```python
from build123d import *

# Parameters (mm, degrees)
EXTRUDE_1_DEPTH     = 900
CUT_EXTRUDE_1_DEPTH = 40


with BuildPart() as part:
    # Эскиз1 → Вытянуть-Тонкостенный1 (new body)
    with BuildSketch(Plane(origin=(0, 0, 0), x_dir=(0, 0, -1), z_dir=(1, 0, 0))):
        with BuildLine():
            Line((-3, 53), (-3, 1))
            ThreePointArc((-3, 1), (-1.828427125, -1.828427125), (1, -3))
            Line((1, -3), (33, -3))
            ThreePointArc((33, -3), (35.828427125, -1.828427125), (37, 1))
            Line((37, 1), (37, 53))
            ThreePointArc((37, 53), (35.828427125, 55.828427125), (33, 57))
            Line((33, 57), (1, 57))
            ThreePointArc((1, 57), (-1.828427125, 55.828427125), (-3, 53))
        make_face()
        with BuildLine():
            Line((0, 53), (0, 1))
            ThreePointArc((0, 1), (0.292893219, 0.292893219), (1, 0))
            Line((1, 0), (33, 0))
            ThreePointArc((33, 0), (33.707106781, 0.292893219), (34, 1))
            Line((34, 1), (34, 53))
            ThreePointArc((34, 53), (33.707106781, 53.707106781), (33, 54))
            Line((33, 54), (1, 54))
            ThreePointArc((1, 54), (0.292893219, 53.707106781), (0, 53))
        make_face(mode=Mode.SUBTRACT)
    extrude(amount=EXTRUDE_1_DEPTH)

    # Эскиз2 → Вырез-Вытянуть1 (cut)
    with BuildSketch(Plane.XY.offset(3)):
        with BuildLine():
            Line((20, 32), (50, 32))
            ThreePointArc((50, 32), (55, 27), (50, 22))
            Line((50, 22), (20, 22))
            ThreePointArc((20, 22), (15, 27), (20, 32))
        make_face()
    extrude(amount=-CUT_EXTRUDE_1_DEPTH, mode=Mode.SUBTRACT)


solid = part.part
```
Geometry: final body of the model. Coordinates: model frame, mm. A direction names the side the tool comes from. Coordinates: 2 decimals unless noted, no trailing zeros. Order: outer loops, then holes, each group sorted by start corner. A loop starts at its lowest first (then second) coordinate and runs counter-clockwise, first axis right, second up. Notation, with made-up numbers: (63.25, -4) - (88.25, -4) arc R33 cw to (88.25, 25) - close; hole circle Ø8 at (-38.5, 70.5). An arc over 180 degrees is marked (long way). Write each question's results on one line, items separated by ' | '.
(1) Set-up query: faces 4 (the face through (444, 27, 0)), 5 (the face through (444, 27, 3)). Return all of +Z, -Z, +X, -X, +Y, -Y with unobstructed straight access to the full face (end or side cutting, diameter ignored); none if empty.
Values found:
face 4: +X, -X | face 5: +Z, +X, -X, +Y, -Y
(2) Section query B-B, the plane z = -14. Return the cut outline in (x, y), plus the area to 3 significant figures.
Values found:
outline: (0, -3) - (900, -3) - (900, 0) - (0, 0) - close; (0, 54) - (900, 54) - (900, 57) - (0, 57) - close | area: 5,400 mm²
(3) Section query C-C, the plane x = 818.5. Return the cut outline in (y, z), plus the area to 3 significant figures.
Values found:
outline: (-3, -33) arc R4 ccw to (1, -37) - (53, -37) arc R4 ccw to (57, -33) - (57, -1) arc R4 ccw to (53, 3) - (1, 3) arc R4 ccw to (-3, -1) - close; hole (0, -33) arc R1 ccw to (1, -34) - (53, -34) arc R1 ccw to (54, -33) - (54, -1) arc R1 ccw to (53, 0) - (1, 0) arc R1 ccw to (0, -1) - close | area: 551 mm²
(4) First-contact query: pin 1 Ø0.9 at (x, z) = (41, -36) entering from +Y; pin 2 Ø1.5 at (x, z) = (29, 2) entering from +Y; pin 3 Ø0.9 at (x, z) = (33, 2) entering from -Y. Flat tips, straight axial feed; report the tip coordinate or a pass-through.
Values found:
pin 1: stops at y = 56.08 | pin 2: stops at y = 56.31 | pin 3: stops at y = -2.08
(5) Line query: line 1 (Z direction, x = 734, y = 21); line 2 (Y direction, x = 351, z = -6). Output: solid intervals per line, ascending. Write a range as [from, to].
Values found:
line 1: z = [-37, -34], [0, 3] | line 2: y = [-3, 0], [54, 57]
(6) Section query A-A, the plane y = 44. Return the cut outline in (x, z), plus the area to 3 significant figures.
Values found:
outline: (0, -37) - (900, -37) - (900, -34) - (0, -34) - close; (0, 0) - (900, 0) - (900, 3) - (0, 3) - close | area: 5,400 mm²
(7) Mould query, pull axis Y, two halves, no side actions, for faces 1 (the face through (0, 27, 1)), 2 (the face through (444, 27, -34)), 3 (the face through (444, -3, -17)). Classes: +Y half, -Y half, draft (parallel to the pull), parting line (faces both ways), or undercut.
Values found:
face 1: draft | face 2: undercut | face 3: -Y half
